Input: part model. Units: mm. Frame: model coordinates. Face numbers are marked on the shaded views. A direction names the side the tool comes from. Coordinates: 2 decimals unless noted, no trailing zeros. Loops run counter-clockwise (first coordinate to the right, second up) from the corner with the lowest first, then second, coordinate; pieces in that order, holes last. Notation, with made-up numbers: (-32.5, -39) - (25.5, -39) arc R10 ccw to (25.5, -22) - close; hole circle Ø11 at (56.25, 2.25). An arc over 180 degrees is marked (long way). Use one line per item in the form item = value.
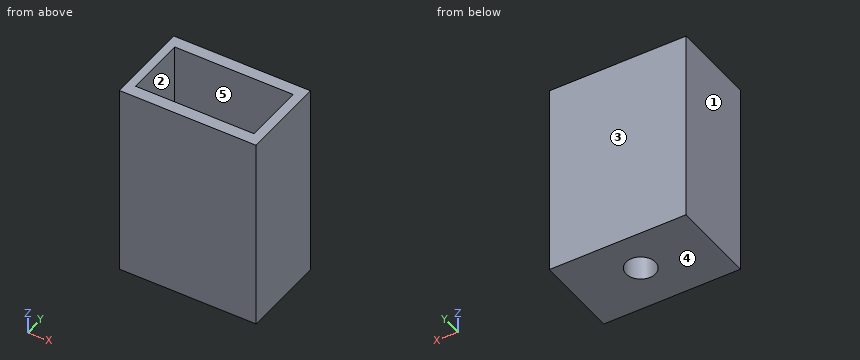
Autodesk Inventor part; units mm, degrees
ref_plane "YZ Plane" through (0, 0, 0) normal (1, 0, 0) x (0, 1, 0)
ref_plane "XZ Plane" through (0, 0, 0) normal (0, 1, 0) x (-1, 0, 0)
ref_plane "XY Plane" through (0, 0, 0) normal (0, 0, 1) x (1, 0, 0)
sketch "Sketch1" plane through (0, 0, 0) normal (0, 0, 1) x (1, 0, 0)
  point P0 (0, 0)
sketch "Sketch2" plane through (0, 0, 0) normal (0, 0, 1) x (1, 0, 0)
  point P0 (0, 0)
sketch "Sketch3" plane through (0, 0, 0) normal (0, 0, 1) x (1, 0, 0)
  line L0 (0, 0) -> (7.112, 0)
  line L1 (7.112, 0) -> (7.112, 4.4704)
  line L2 (7.112, 4.4704) -> (0, 4.4704)
  line L3 (0, 4.4704) -> (0, 0)
  dimension "d0" = 7.112
  dimension "d1" = 4.4704
extrude "Extrusion1" add sketch "Sketch3" along normal blind 10.16
sketch "Sketch4" plane through (0, 0, 10.16) normal (0, 0, 1) x (1, 0, 0)
  line L0 (0.4347, 3.8467) -> (6.6067, 3.8467)
  line L1 (6.6067, 3.8467) -> (6.6067, 0.6302)
  line L2 (6.6067, 0.6302) -> (0.4347, 0.6302)
  line L3 (0.4347, 0.6302) -> (0.4347, 3.8467)
  point P0 (0, 0)
extrude "Extrusion2" cut sketch "Sketch4" against normal blind 7.62
sketch "Sketch5" plane through (0, 0, 0) normal (0, 0, -1) x (-1, 0, 0)
  circle A0 centre (-3.6638, 2.4113) radius 0.7685
  point P0 (0, 0)
extrude "Extrusion3" cut sketch "Sketch5" against normal blind 2.54
properties part number "dc motor"
Q1. Cut plane A-A, the plane z = 9. Return loops of the section in (x, y), then the cut area to 3 significant figures.
Check values:
outline = (0, 0) - (7.11, 0) - (7.11, 4.47) - (0, 4.47) - close; hole (0.43, 0.63) - (6.61, 0.63) - (6.61, 3.85) - (0.43, 3.85) - close
area = 11.9 mm²
Q2. Ray query, line 1 along Y through (x, z) = (2.5, 8.5); line 2 along X through (y, z) = (3.45, 4); line 3 along Z through (x, y) = (2, 1.3). Return the intervals inside material, ascending. Write a range as [from, to].
Check values:
line_1 = [0, 0.63], [3.85, 4.47]
line_2 = [0, 0.43], [6.61, 7.11]
line_3 = [0, 2.54]
Q3. Cut plane B-B, the plane y = 2. Return loops of the section in (x, z), then the cut area to 3 significant figures.
Check values:
outline = (0, 0) - (3.01, 0) - (3.01, 2.54) - (0.43, 2.54) - (0.43, 10.16) - (0, 10.16) - close; (4.31, 0) - (7.11, 0) - (7.11, 10.16) - (6.61, 10.16) - (6.61, 2.54) - (4.31, 2.54) - close
area = 21.9 mm²
Q4. Pull-direction query (X, two-part tool) for the marked faces 1, 2 and 3; classes: pulls with the +X half, pulls with the -X half, needs draft (parallel to the pull), parting line crosses it, or undercut.
Check values:
face_1 = pulls with the -X half
face_2 = undercut
face_3 = needs draft
Q5. Cut plane D-D, the plane y = 0.95. Return loops of the section in (x, z).
Check values:
outline = (0, 0) - (7.11, 0) - (7.11, 10.16) - (6.61, 10.16) - (6.61, 2.54) - (0.43, 2.54) - (0.43, 10.16) - (0, 10.16) - close
Q6. Set-up query: the marked faces 4 and 5. Return all of +Z, -Z, +X, -X, +Y, -Y with unobstructed straight access to the full face (end or side cutting, diameter ignored); none if empty.
Check values:
face_4 = -Z, +X, -X, +Y, -Y
face_5 = +Z
Q7. First-contact query: P1, Ø1.9, axis at x = 3.5, z = 6.5, coming from the -Y side. Flat tip, straight axial feed; report the tip coordinate or a pass-through.
Check values:
P1 = 0
Q8. Cut plane C-C, the plane x = 3.75. Return loops of the section in (y, z).
Check values:
outline = (0, 0) - (1.65, 0) - (1.65, 2.54) - (0.63, 2.54) - (0.63, 10.16) - (0, 10.16) - close; (3.17, 0) - (4.47, 0) - (4.47, 10.16) - (3.85, 10.16) - (3.85, 2.54) - (3.17, 2.54) - close
